from build123d import *

# Parameters (mm, degrees)
SKETCH2_R           = 1.5
BOSS_EXTRUDE1_DEPTH = 0.5
FILLET1_R           = 0.3


with BuildPart() as part:
    # Sketch1 → Revolve1 (revolve)
    with BuildSketch(Plane.XY, mode=Mode.PRIVATE) as revolve1_sk:
        Polygon((0, 0), (6.5, 0), (4.5, 2), (4.5, 10), (0, 10), align=None)
    revolve(revolve1_sk.sketch.rotate(Axis((0, 10, 0), (0, -1, 0)), 180), axis=Axis((0, 10, 0), (0, -1, 0)))  # turned: the seam where the file's is

    # Sketch2 → Boss-Extrude1 (add)
    with BuildSketch(Plane.XZ):
        with Locations(Location((4, 0, 0), (0, 0, 180))):  # turned: the seam where the file's is
            Circle(SKETCH2_R)
    extrude(amount=BOSS_EXTRUDE1_DEPTH)

    # Fillet1
    fillet1_edges = [part.edges().sort_by_distance(p)[0] for p in [
        (5.5, -0.5, 0),
    ]]
    fillet(fillet1_edges, radius=FILLET1_R)


solid = part.part
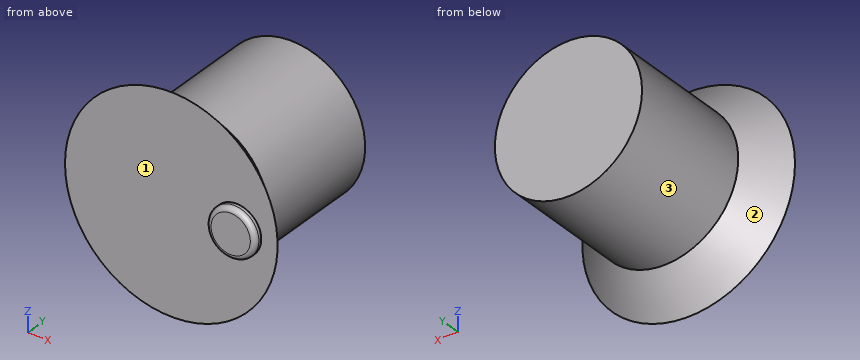
Model file for the job. Use its own axes, mm. Face numbers are marked on the shaded views. Coordinates: 2 decimals unless noted, no trailing zeros. Order: outer loops, then holes, each group sorted by start corner. A loop starts at its lowest first (then second) coordinate and runs counter-clockwise, first axis right, second up. Notation, with made-up numbers: (6, -27) -> (39, -27) arc R12 ccw to (39, -11) -> close; hole circle Ø9 at (89.5, 27). An arc over 180 degrees is marked (long way). Return JSON: item names as keys, results as strings. Group by question number.
Item 1: Flat gauge pins, fed straight in: P1, Ø1.5, axis at x = 1, z = -2.5, coming from the -Y side; P2, Ø3, axis at x = 4, y = 5, coming from the -Z side; P3, Ø2, axis at y = 6.5, z = -2.5, coming from the +X side. Where does each tip first touch, or does it go through?
Item 2: Wall check: line 1 along Y through (x, z) = (-1.5, 2.75); line 2 along Z through (x, y) = (2.75, 9); line 3 along X through (y, z) = (8.5, -2.5). Give the ranges that are in metal, low to high. Write a range as [from, to].
Item 3: Saw through at C-C on y = 7.25. Write the cut outline in (x, z).
Item 4: Saw through at A-A on z = 0. Write the cut outline in (x, y).
Item 5: Pull direction Y, two halves, no side cores. Call the marked faces 1, 2 and 3: pulls with the +Y half, pulls with the -Y half, needs draft (parallel to the pull), parting line crosses it, or undercut.
Item 6: Saw through at B-B on x = 0. Write the cut outline in (y, z), then the cut area to 3 significant figures.
Values found:
{
 "1": {"P1": "stops at y = 0", "P2": "stops at z = -3.74", "P3": "stops at x = 4.24"},
 "2": {"line 1": "y = [0, 10]", "line 2": "z = [-3.56, 3.56]", "line 3": "x = [-3.74, 3.74]"},
 "3": {"outline": "circle Ø9 at (0, 0)"},
 "4": {"outline": "(-6.5, 0) -> (2.5, 0) -> (2.5, -0.2) arc R0.3 ccw to (2.8, -0.5) -> (5.2, -0.5) arc R0.3 ccw to (5.5, -0.2) -> (5.5, 0) -> (6.5, 0) -> (4.5, 2) -> (4.5, 10) -> (-4.5, 10) -> (-4.5, 2) -> close"},
 "5": {"face 1": "pulls with the -Y half", "face 2": "pulls with the +Y half", "face 3": "needs draft"},
 "6": {"outline": "(0, -6.5) -> (2, -4.5) -> (10, -4.5) -> (10, 4.5) -> (2, 4.5) -> (0, 6.5) -> close", "area": "94.0 mm2"}
}
